Can you work these out from the drawing? Everything is in mm from the part's minimum corner. A direction names the side the tool comes from. Round coordinates to 2 decimals unless told otherwise and drop trailing zeros. Loops run counter-clockwise (first coordinate to the right, second up) from the corner with the lowest first, then second, coordinate; pieces in that order, holes last. Notation, with made-up numbers: (-7, 27) - (45, 27) arc R25 cw to (45, 46) - close; hole circle Ø6 at (21, 62). An arc over 180 degrees is marked (long way). Return JSON: item names as keys, results as strings. Group by question number.
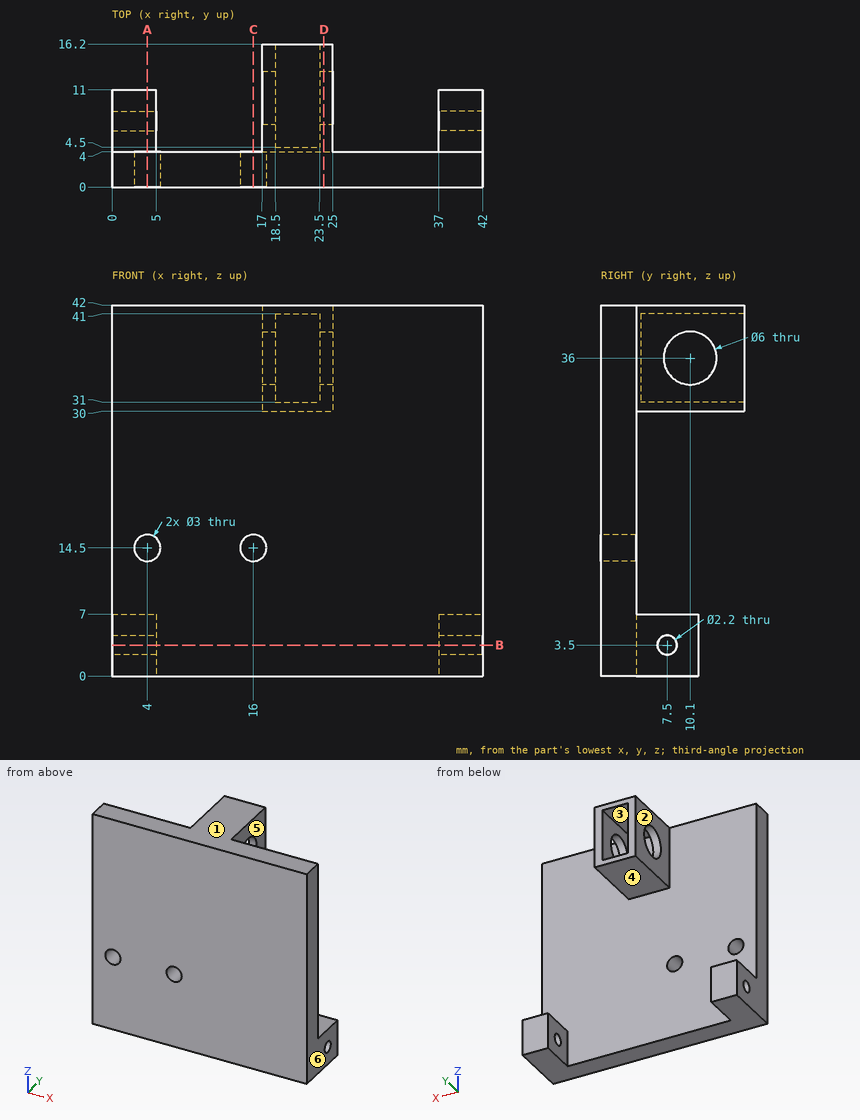
Q1. Please list where these lines run through material, in increasing order: line 1 (X direction, y = 4.5, z = 6); line 2 (X direction, y = 8.75, z = 32); line 3 (Y direction, x = 24.1, z = 36).
Q2. If we mould it in two halves opening along X, with no side actions, what happens to the marked faces 1, 2 and 3? For each: +X half, -X half, draft (parallel to the pull), parting line (faces both ways), or undercut.
Q3. Imagine slicing it at B-B, the plane z = 3.5. List the corners of the cut face in (x, y) for me, and give its area (3 significant figures).
Q4. For the marked faces 4, 5 and 6, which set-ups out of +Z, -Z, +X, -X, +Y, -Y let a thin tool reach every point of the face, with its end or its side?
Q5. Will these pins go through, and if not, where does the flat tip stop? pin 1 Ø5 at (x, z) = (16, 14.5) entering from +Y; pin 2 Ø7 at (y, z) = (10.1, 36) entering from -X; pin 3 Ø4 at (x, z) = (37, 5.5) entering from +Y.
Q6. Imagine slicing it at A-A, the plane x = 4. List the corners of the cut face in (y, z) for me, and give its area (3 significant figures).
Q7. Imagine slicing it at D-D, the plane x = 24. List the corners of the cut face in (y, z) for me.
Q8. Imagine slicing it at C-C, the plane x = 16. List the corners of the cut face in (y, z) for me.
Output values:
{
 "1": {"line 1": "x = 0 to 5, 37 to 42", "line 2": "x = 17 to 18.5, 23.5 to 25", "line 3": "y = 0 to 7.1, 13.1 to 16.2"},
 "2": {"face 1": "draft", "face 2": "-X half", "face 3": "undercut"},
 "3": {"outline": "(0, 0) - (42, 0) - (42, 6.4) - (37, 6.4) - (37, 4) - (5, 4) - (5, 6.4) - (0, 6.4) - close; (0, 8.6) - (5, 8.6) - (5, 11) - (0, 11) - close; (37, 8.6) - (42, 8.6) - (42, 11) - (37, 11) - close", "area": "216 mm^2"},
 "4": {"face 4": "-Z, +X, -X, +Y", "face 5": "+Z, -Z, +X, +Y", "face 6": "+Z, -Z, +X, +Y, -Y"},
 "5": {"pin 1": "stops at y = 4", "pin 2": "stops at x = 17", "pin 3": "stops at y = 11"},
 "6": {"outline": "(0, 0) - (11, 0) - (11, 7) - (4, 7) - (4, 13) - (0, 13) - close; (0, 16) - (4, 16) - (4, 42) - (0, 42) - close; hole circle Ø2.2 at (7.5, 3.5)", "area": "201 mm^2"},
 "7": {"outline": "(0, 0) - (4, 0) - (4, 30) - (16.2, 30) - (16.2, 42) - (0, 42) - close; hole circle Ø6 at (10.1, 36)"},
 "8": {"outline": "(0, 0) - (4, 0) - (4, 13) - (0, 13) - close; (0, 16) - (4, 16) - (4, 42) - (0, 42) - close"}
}
